Geometry: see drawing. Coordinates: mm, zero at the bounding-box minimum. Give positions to 0.01 mm unless a question says otherwise; leave off trailing zeros. Order: outer loops, then holes, each group sorted by start corner. A loop starts at its lowest first (then second) coordinate and runs counter-clockwise, first axis right, second up. Notation, with made-up numbers: (38, 9) -> (89, 9) arc R21 ccw to (89, 38) -> close; hole circle Ø3 at (16, 88). An arc over 180 degrees is marked (long way). One line per item, written item: value. Start each with the question number.
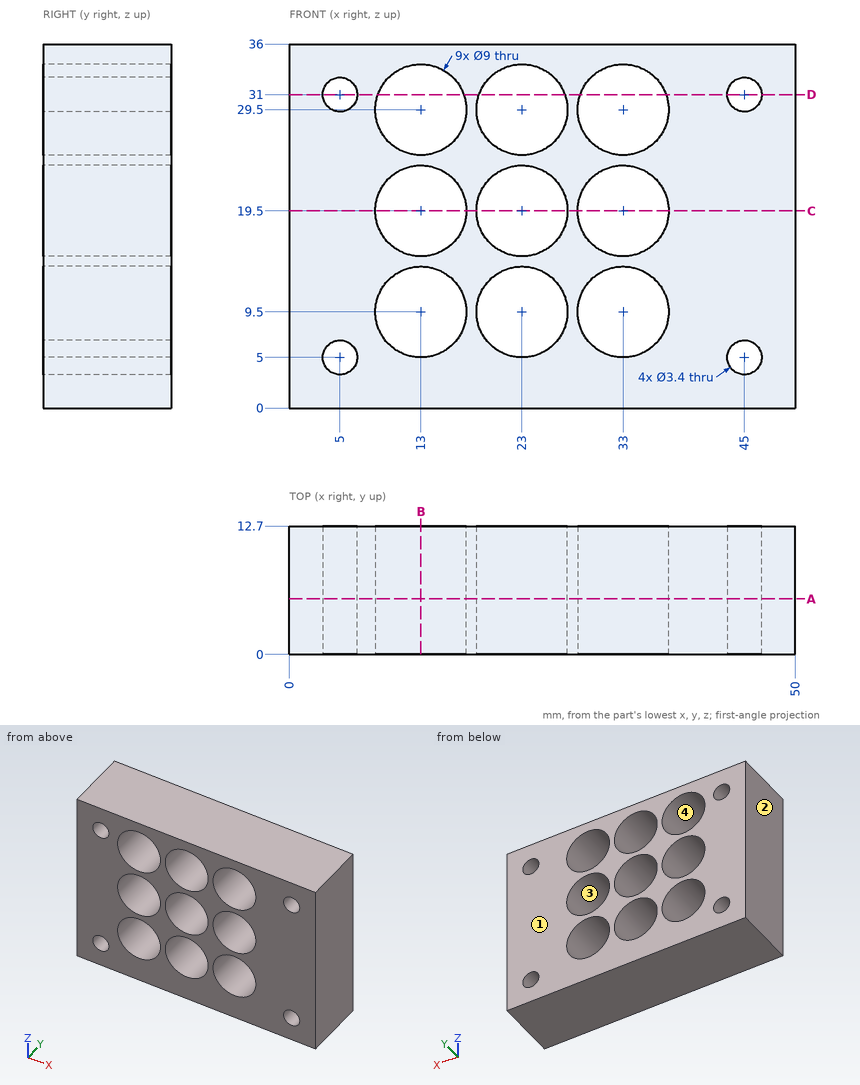
1. Cut plane C-C, the plane z = 19.5. Return loops of the section in (x, y).
2. Cut plane A-A, the plane y = 5.5. State how many separate pieces and enclosed holes the cut face has, then the cut area to 3 significant figures.
3. Cut plane B-B, the plane x = 13. Return loops of the section in (y, z), then the cut area to 3 significant figures.
4. Cut plane D-D, the plane z = 31. Return loops of the section in (x, y).
5. Draft query along X for the marked faces 1, 2, 3 and 4. Return one class per face: pulls with the +X half, pulls with the -X half, needs draft (parallel to the pull), parting line crosses it, or undercut.
6. Material intervals for L1, parallel to Z at x = 33, y = 9.75; L2, parallel to Z at x = 5, y = 8.75; L3, parallel to X at y = 8, z = 9.5, sorted ascending. Write a range as [from, to].
Answers follow:
1. outline: (0, 0) -> (8.5, 0) -> (8.5, 12.7) -> (0, 12.7) -> close; (17.5, 0) -> (18.5, 0) -> (18.5, 12.7) -> (17.5, 12.7) -> close; (27.5, 0) -> (28.5, 0) -> (28.5, 12.7) -> (27.5, 12.7) -> close; (37.5, 0) -> (50, 0) -> (50, 12.7) -> (37.5, 12.7) -> close
2. separate pieces: 1
2. enclosed holes: 13
2. area: 1,190 mm²
3. outline: (0, 0) -> (12.7, 0) -> (12.7, 5) -> (0, 5) -> close; (0, 14) -> (12.7, 14) -> (12.7, 15) -> (0, 15) -> close; (0, 24) -> (12.7, 24) -> (12.7, 25) -> (0, 25) -> close; (0, 34) -> (12.7, 34) -> (12.7, 36) -> (0, 36) -> close
3. area: 114 mm²
4. outline: (0, 0) -> (3.3, 0) -> (3.3, 12.7) -> (0, 12.7) -> close; (6.7, 0) -> (8.76, 0) -> (8.76, 12.7) -> (6.7, 12.7) -> close; (17.24, 0) -> (18.76, 0) -> (18.76, 12.7) -> (17.24, 12.7) -> close; (27.24, 0) -> (28.76, 0) -> (28.76, 12.7) -> (27.24, 12.7) -> close; (37.24, 0) -> (43.3, 0) -> (43.3, 12.7) -> (37.24, 12.7) -> close; (46.7, 0) -> (50, 0) -> (50, 12.7) -> (46.7, 12.7) -> close
5. face 1: needs draft
5. face 2: pulls with the -X half
5. face 3: undercut
5. face 4: undercut
6. L1: z = [0, 5], [14, 15], [24, 25], [34, 36]
6. L2: z = [0, 3.3], [6.7, 29.3], [32.7, 36]
6. L3: x = [0, 8.5], [17.5, 18.5], [27.5, 28.5], [37.5, 50]
